```python
from build123d import *

# Parameters (mm, degrees)
EXTRUDE_1_DEPTH        = 276
EXTRUDE_1_2_DEPTH      = 276
EXTRUDE_2_DEPTH        = 12
PATTERN_LINEAR_1_COUNT = 2
PATTERN_LINEAR_1_PITCH = 288
SKETCH_3_W             = 276
SKETCH_3_H             = 12
EXTRUDE_3_DEPTH        = 1000
SKETCH_4_W             = 400
SKETCH_4_H             = 300
EXTRUDE_4_DEPTH        = 12
SKETCH_5_W             = 150
SKETCH_5_H             = 12
EXTRUDE_5_DEPTH        = 100
SKETCH_6_R             = 25
CUT_EXTRUDE_1_DEPTH    = 635.502955076
SKETCH_7_R             = 25
CUT_EXTRUDE_2_DEPTH    = 650.458235763
SKETCH_8_W             = 100
SKETCH_8_H             = 276
CUT_EXTRUDE_3_DEPTH    = 645.003105583


with BuildPart() as part:
    # Sketch 1 → Extrude 1 (new body)
    with BuildSketch(Plane.XY):
        Polygon((-300, 0), (-200, 0), (-200, -150), (-212, -150), (-212, -12), (-300, -12), align=None)
    extrude(amount=EXTRUDE_1_DEPTH)



with BuildPart() as body_2:
    # Sketch 1 → Extrude 1 2 (new body)
    with BuildSketch(Plane.XY):
        Polygon((300, 0), (200, 0), (200, -150), (212, -150), (212, -12), (300, -12), align=None)
    extrude(amount=EXTRUDE_1_2_DEPTH)


with BuildPart() as part_1:
    add(part.part)

    add(body_2.part)  # Extrude 2 merges body 2
    # Sketch 2 → Extrude 2 (add)
    with BuildSketch(Plane.XY.offset(276)):
        Polygon((-500, 12), (500, 12), (500, -88), (200, -175), (-200, -175), (-500, -88), align=None)
    extrude_2 = extrude(amount=EXTRUDE_2_DEPTH)

    # Pattern Linear 1: Extrude 2 ×2
    with Locations(*[(0, 0, -i * PATTERN_LINEAR_1_PITCH) for i in range(1, PATTERN_LINEAR_1_COUNT)]):
        add(extrude_2)

    # Sketch 3 → Extrude 3 (add)
    with BuildSketch(Plane(origin=(500, 0, 0), x_dir=(0, 0, -1), z_dir=(1, 0, 0))):
        with Locations((-138, 6)):
            Rectangle(SKETCH_3_W, SKETCH_3_H)
    extrude(amount=-EXTRUDE_3_DEPTH)

    # Sketch 4 → Extrude 4 (add)
    with BuildSketch(Plane.XZ.offset(175)):
        with Locations((0, 138)):
            Rectangle(SKETCH_4_W, SKETCH_4_H)
    extrude(amount=EXTRUDE_4_DEPTH)

    # Sketch 5 → Extrude 5 (add)
    with BuildSketch(Plane(origin=(0, -187, 0), x_dir=(-1, 0, 0), z_dir=(0, -1, 0))):
        with Locations((0, -247)):
            Rectangle(SKETCH_5_W, SKETCH_5_H)
        with Locations((0, -29)):
            Rectangle(SKETCH_5_W, SKETCH_5_H)
    extrude(amount=EXTRUDE_5_DEPTH)

    # Sketch 6 → Cut-Extrude 1 (cut, through all)
    with BuildSketch(Plane.XY.offset(253)):
        with Locations((0, -238)):
            Circle(SKETCH_6_R)
        with BuildLine():
            Line((75, -211), (75, -287))
            Line((75, -287), (-75, -287))
            Line((-75, -287), (-75, -211))
            ThreePointArc((-75, -211), (0, -286), (75, -211))
        make_face()
    extrude(amount=-CUT_EXTRUDE_1_DEPTH, mode=Mode.SUBTRACT)

    # Sketch 7 → Cut-Extrude 2 (cut, through all)
    with BuildSketch(Plane.XY.offset(288)):
        with Locations((-362.5, -38)):
            Circle(SKETCH_7_R)
        with Locations((362.5, -38)):
            Circle(SKETCH_7_R)
        with Locations((0, -38)):
            Circle(SKETCH_7_R)
    extrude(amount=-CUT_EXTRUDE_2_DEPTH, mode=Mode.SUBTRACT)

    # Sketch 8 → Cut-Extrude 3 (cut, through all)
    with BuildSketch(Plane.XZ):
        with Locations((362.5, 138)):
            Rectangle(SKETCH_8_W, SKETCH_8_H)
        with Locations((-362.5, 138)):
            Rectangle(SKETCH_8_W, SKETCH_8_H)
        with Locations((0, 138)):
            Rectangle(SKETCH_8_W, SKETCH_8_H)
    extrude(amount=-CUT_EXTRUDE_3_DEPTH, mode=Mode.SUBTRACT)


solid = part_1.part
```
Model file for the job. Use its own axes, mm. A direction names the side the tool comes from. Coordinates: 2 decimals unless noted, no trailing zeros. Loops run counter-clockwise (first coordinate to the right, second up) from the corner with the lowest first, then second, coordinate; pieces in that order, holes last. Notation, with made-up numbers: M -19.75,2.25 L 16.25,2.25 A11 cw 16.25,21.25 Z; hole C -7.5,81 d8. An arc over 180 degrees is marked long. Use CSV: the item, a comma, the result in double quotes. Start each with the question number.
1. Band-saw the part on C-C, the plane x = 171. List the corners of the cut face in (y, z), then the cut area to 3 significant figures.
2. Two-plate mould, pull along Y, no slides. Class faces 1 (the flat face through (-347.9, -132.11, 281.92)), 2 (the flat face through (212, -82, 136)), 3 (the cylindrical face through (-3.255, -213.213, 29.084)): pulls with the +Y half, pulls with the -Y half, needs draft (parallel to the pull), parting line crosses it, or undercut.
3. Probe probe 1 along X at (y, z) = (-76.5, 28.5); probe 2 along Z at (x, y) = (50.5, -110.5); probe 3 along Y at (x, z) = (107, 63). List the from-to ranges inside material, lowest first. Write a range as [from, to].
4. Flat gauge pins, fed straight in: pin 1 (12 mm diameter, centred on x = 73, y = -206.5, fed in from -Z); pin 2 (6 mm diameter, centred on x = -304, z = 104.5, fed in from -Y); pin 3 (8 mm diameter, centred on y = -144, z = 60, fed in from -X). Where does each tip first touch, or does it go through?
5. Tool access for faces 4 (the flat face through (-212, -82, 136)), 5 (the flat face through (-16, -214, 23)), 6 (the flat face through (-3, -175, 140)), 7 (the flat face through (7, -80, 0)): list every direction of +Z, -Z, +X, -X, +Y, -Y with a clear straight run to the whole face (end or side of a thin tool).
6. Band-saw the part on A-A, the plane x = 0. Give the number of separate pieces and of enclosed holes in the cut face, then the cut area to 3 significant figures.
7. Band-saw the part on D-D, the plane x = -362.5. List the corners of the cut face in (y, z) (3 decimals).
Entries:
1,outline,"M -187,-12 L 12,-12 L 12,288 L -187,288 Z; hole M -175,0 L 0,0 L 0,276 L -175,276 Z"
1,area,"11,400 mm2"
2,face 1,"pulls with the -Y half"
2,face 2,"needs draft"
2,face 3,"undercut"
3,probe 1,"x = [-212, -200], [200, 212]"
3,probe 2,"z = [-12, 0], [276, 288]"
3,probe 3,"y = [-187, -175], [0, 12]"
4,pin 1,"stops at z = 23"
4,pin 2,"stops at y = 0"
4,pin 3,"stops at x = -212"
5,face 4,"-X, -Y"
5,face 5,"-Z, +X, -X, -Y"
5,face 6,"+X, -X"
5,face 7,"none"
6,separate pieces,"5"
6,enclosed holes,"0"
6,area,"8,060 mm2"
7,outline,"M -127.875,-12 L -63,-12 L -63,0 L -127.875,0 Z; M -127.875,276 L -63,276 L -63,288 L -127.875,288 Z; M -13,-12 L 12,-12 L 12,0 L -13,0 Z; M -13,276 L 12,276 L 12,288 L -13,288 Z"
